Build history of the part. All positions in model axes, mm. Give positions to 0.01 mm unless a question says otherwise; leave off trailing zeros. Write each loop counter-clockwise with the first axis right and the second up, starting at its lowest first coordinate (ties: lowest second). Pieces come first, ordered by that corner, then holes.
Autodesk Inventor part; units mm, degrees
ref_plane "YZ Plane" through (0, 0, 0) normal (1, 0, 0) x (0, 1, 0)
ref_plane "XZ Plane" through (0, 0, 0) normal (0, 1, 0) x (-1, 0, 0)
ref_plane "XY Plane" through (0, 0, 0) normal (0, 0, 1) x (1, 0, 0)
sketch "Sketch1" plane through (0, 0, 0) normal (0, 1, 0) x (-1, 0, 0)
  circle A0 centre (0, 0) radius 12.75
  line L0 (13, 15) -> (-13, 15)
  line L1 (-15, 13) -> (-15, -13)
  line L2 (-13, -15) -> (13, -15)
  line L3 (15, -13) -> (15, 13)
  line L4 (15, 15) -> (-15, -15) construction
  line L5 (-15, 15) -> (15, -15) construction
  arc A1 (15, 13) -> (13, 15) centre (13, 13) ccw
  arc A2 (13, -15) -> (15, -13) centre (13, -13) ccw
  arc A3 (-15, -13) -> (-13, -15) centre (-13, -13) ccw
  arc A4 (-13, 15) -> (-15, 13) centre (-13, 13) ccw
  dimension "d0" = 25.5
  dimension "d1" = 30
  dimension "d2" = 30
  dimension "d3" = 2
extrude "Extrusion1" add sketch "Sketch1" along normal blind 5
sketch "Sketch2" plane through (0, 5, 0) normal (0, 1, 0) x (1, 0, 0)
  circle A0 centre (0, 0) radius 12.75
  line L0 (-13, -15) -> (13, -15)
  arc A1 (13, -15) -> (15, -13) centre (13, -13) ccw
  line L1 (15, -13) -> (15, 13)
  arc A2 (15, 13) -> (13, 15) centre (13, 13) ccw
  line L2 (13, 15) -> (-13, 15)
  arc A3 (-13, 15) -> (-15, 13) centre (-13, 13) ccw
  line L3 (-15, 13) -> (-15, -13)
  arc A4 (-15, -13) -> (-13, -15) centre (-13, -13) ccw
  line L4 (12, 12) -> (-12, 12)
  line L5 (-12, 12) -> (-12, -12)
  line L6 (-12, -12) -> (12, -12)
  line L7 (12, -12) -> (12, 12)
  line L8 (12, 12) -> (-12, -12) construction
  line L9 (-12, 12) -> (12, -12) construction
  dimension "d6" = 24
  dimension "d7" = 24
  dimension "d15" = 30
hole "Hole1" at (-12, 5, -12) at (12, 5, -12) at (12, 5, 12) at (-12, 5, 12) direction (0, -1, 0) diameter 2.9 depth 24 tip angle 118
properties part number "100_Adapter_Waveplate"
(1) Drop a flat-ended pin along its axis: pin 1 (5 mm diameter, centred on x = -9.5, z = 5.5, fed in from -Y). Give the stop position or say it passes through.
(2) Mould opens along Z. For faces 1 (the face through (14, 0, 0)), 2 (the face through (-14.43, 2.46, -14.4)), 3 (the face through (-11.12, 2.46, 10.85)), 4 (the face through (12.88, 2.46, 10.85)) say: +Z half, -Z half, draft (parallel to the pull), parting line (faces both ways), or undercut.
(3) Saw through at A-A, the plane z = 0. List the corners of the cut face in (x, y).
(4) Saw through at C-C, the plane y = 1.2. List the corners of the cut face in (x, z), plus the area to 3 significant figures.
(5) Probe line 1 (Z direction, x = -11, y = 1.6); line 2 (Z direction, x = 0, y = 3.8); line 3 (X direction, y = 4.2, z = 3.5). List the from-to ranges inside material, lowest first.
(6) Saw through at B-B, the plane x = 0. List the corners of the cut face in (y, z).
(7) Saw through at D-D, the plane x = 11.5. List the corners of the cut face in (y, z), plus the area to 3 significant figures.
Computed values:
1. pin 1: stops at y = 0
2. face 1: draft
2. face 2: -Z half
2. face 3: undercut
2. face 4: undercut
3. outline: (-15, 0) - (-12.75, 0) - (-12.75, 5) - (-15, 5) - close; (12.75, 0) - (15, 0) - (15, 5) - (12.75, 5) - close
4. outline: (-15, -13) arc R2 ccw to (-13, -15) - (13, -15) arc R2 ccw to (15, -13) - (15, 13) arc R2 ccw to (13, 15) - (-13, 15) arc R2 ccw to (-15, 13) - close; hole circle Ø2.9 at (-12, -12); hole circle Ø2.9 at (-12, 12); hole circle Ø25.5 at (0, 0); hole circle Ø2.9 at (12, -12); hole circle Ø2.9 at (12, 12)
4. area: 359 mm2
5. line 1: z = -15 to -13.05, -10.95 to -6.45, 6.45 to 10.95, 13.05 to 15
5. line 2: z = -15 to -12.75, 12.75 to 15
5. line 3: x = -15 to -12.26, 12.26 to 15
6. outline: (0, -15) - (5, -15) - (5, -12.75) - (0, -12.75) - close; (0, 12.75) - (5, 12.75) - (5, 15) - (0, 15) - close
7. outline: (0, -15) - (5, -15) - (5, -13.36) - (0, -13.36) - close; (0, -10.64) - (5, -10.64) - (5, -5.51) - (0, -5.51) - close; (0, 5.51) - (5, 5.51) - (5, 10.64) - (0, 10.64) - close; (0, 13.36) - (5, 13.36) - (5, 15) - (0, 15) - close
7. area: 67.7 mm2
